Autodesk Inventor part; units mm, degrees
ref_plane "作業平面1" through (0, 80, 0) normal (0, 1, 0) x (1, 0, 0)
ref_plane "YZ Plane" through (0, 0, 0) normal (1, 0, 0) x (0, 1, 0)
ref_plane "XZ Plane" through (0, 0, 0) normal (0, 1, 0) x (-1, 0, 0)
sketch "スケッチ1" plane through (0, 0, 0) normal (0, 1, 0) x (-1, 0, 0)
  circle A0 centre (0, 0) radius 4
  dimension "d0" = 8
extrude "押し出し1" add sketch "スケッチ1" along normal blind 160
ref_plane "作業平面1" through (0, 80, 0) normal (0, 1, 0) x (1, 0, 0)
sketch "スケッチ2" plane through (0, 80, 0) normal (0, 1, 0) x (1, 0, 0)
  circle A0 centre (0, 0) radius 4
  circle A1 centre (0, 0) radius 5
  dimension "d3" = 10
extrude "押し出し2" add sketch "スケッチ2" along normal blind 25.9 and the other way blind 25.9 contours A0 | A1
sketch "スケッチ3" plane through (0, 80, 0) normal (0, 1, 0) x (1, 0, 0)
  point P0 (0, 0)
properties part number "elbow_shaft2"
Can you work these out from the model? Positions are in its coordinate system, mm. A direction names the side the tool comes from. Give positions to 0.01 mm unless a question says otherwise; leave off trailing zeros. Order: outer loops, then holes, each group sorted by start corner. A loop starts at its lowest first (then second) coordinate and runs counter-clockwise, first axis right, second up. Notation, with made-up numbers: M 7,62 L 37,62 A18 ccw 37,96 Z; hole C 72,-39 d5. An arc over 180 degrees is marked long. Use a Markdown table: item, result. Add a question column.
Item 1: Suppose I cut it at B-B (x = 0). List the corners of the cut face in (y, z) for me.
Item 2: For faces 1 (the flat face through (0, 160, 0)), 2 (the cylindrical face through (0.867, 26.671, 3.905)), 3 (the cylindrical face through (0.867, 132.571, 3.905)), which set-ups out of +Z, -Z, +X, -X, +Y, -Y let a thin tool reach every point of the face, with its end or its side?
Item 3: Will these pins go through, and if not, where does the flat tip stop? pin 1 (1.5 mm diameter, centred on y = 117, z = 3, fed in from +X); pin 2 (6 mm diameter, centred on y = 137, z = 3, fed in from +X); pin 3 (6 mm diameter, centred on x = -1.5, y = 122, fed in from -Z).
Item 4: Suppose I cut it at D-D (y = 121.5). List the corners of the cut face in (x, z) for me, then the cut area to 3 significant figures.
Item 5: Suppose I cut it at C-C (y = 56). List the corners of the cut face in (x, z) for me, then the cut area to 3 significant figures.
Item 6: Suppose I cut it at A-A (z = 0). List the corners of the cut face in (x, y) for me, then the cut area to 3 significant figures.
Item 7: If I drill on L1, parallel to Y at x = 4, z = 1.5; L2, parallel to X at y = 71.5, z = 0.25; L3, parallel to X at y = 45, z = -0.25, over which ranges is the centre line in solid material (lowest first)? Write a range as [from, to].
Answer sheet:
| question | item | result |
|---|---|---|
| 1 | outline | M 0,-4 L 54.1,-4 L 54.1,-5 L 105.9,-5 L 105.9,-4 L 160,-4 L 160,4 L 105.9,4 L 105.9,5 L 54.1,5 L 54.1,4 L 0,4 Z |
| 2 | face 1 | +Z, -Z, +X, -X, +Y |
| 2 | face 2 | -Y |
| 2 | face 3 | +Y |
| 3 | pin 1 | stops at x = 3.31 |
| 3 | pin 2 | stops at x = 4 |
| 3 | pin 3 | stops at z = -4 |
| 4 | outline | C 0,0 d8 |
| 4 | area | 50.3 mm² |
| 5 | outline | C 0,0 d10 |
| 5 | area | 78.5 mm² |
| 6 | outline | M -5,54.1 L -4,54.1 L -4,0 L 4,0 L 4,54.1 L 5,54.1 L 5,105.9 L 4,105.9 L 4,160 L -4,160 L -4,105.9 L -5,105.9 Z |
| 6 | area | 1,380 mm² |
| 7 | L1 | y = [54.1, 105.9] |
| 7 | L2 | x = [-4.99, 4.99] |
| 7 | L3 | x = [-3.99, 3.99] |
